Geometry check sheet. Reference: the model listing, model coordinates, mm. Face numbers are marked on the shaded views. A direction names the side the tool comes from. Coordinates: 2 decimals unless noted, no trailing zeros. Loops run counter-clockwise (first coordinate to the right, second up) from the corner with the lowest first, then second, coordinate; pieces in that order, holes last. Notation, with made-up numbers: M 1.25,39 L 20.25,39 A13 cw 20.25,60 Z; hole C 50,-27 d4. An arc over 180 degrees is marked long. One line per question, with ' | ' between items. Start each with the question number.
from build123d import *

# Parameters (mm, degrees)
F1_DEPTH = 18
F2_DEPTH = 16
F3_DEPTH = 14
F4_DEPTH = 12
F5_DEPTH = 10
F6_DEPTH = 8
F7_DEPTH = 6
F8_DEPTH = 4
F9_DEPTH = 2


with BuildPart() as f1:
    # F0 (on Top) → F1 (new body)
    with BuildSketch(Plane.XY):
        with BuildLine():
            Line((-5, 0), (-4.5, 0))
            ThreePointArc((-4.5, 0), (0, 4.5), (4.5, 0))
            Line((4.5, 0), (5, 0))
            ThreePointArc((5, 0), (0, 5), (-5, 0))
        make_face()
    extrude(amount=F1_DEPTH)

    # F0 (on Top) → F2 (join)
    with BuildSketch(Plane.XY):
        with BuildLine():
            Line((-4.5, 0), (-4, 0))
            ThreePointArc((-4, 0), (0, 4), (4, 0))
            Line((4, 0), (4.5, 0))
            ThreePointArc((4.5, 0), (0, 4.5), (-4.5, 0))
        make_face()
    extrude(amount=F2_DEPTH)

    # F0 (on Top) → F3 (join)
    with BuildSketch(Plane.XY):
        with BuildLine():
            Line((-4, 0), (-3.5, 0))
            ThreePointArc((-3.5, 0), (0, 3.5), (3.5, 0))
            Line((3.5, 0), (4, 0))
            ThreePointArc((4, 0), (0, 4), (-4, 0))
        make_face()
    extrude(amount=F3_DEPTH)

    # F0 (on Top) → F4 (join)
    with BuildSketch(Plane.XY):
        with BuildLine():
            Line((-3.5, 0), (-3, 0))
            ThreePointArc((-3, 0), (0, 3), (3, 0))
            Line((3, 0), (3.5, 0))
            ThreePointArc((3.5, 0), (0, 3.5), (-3.5, 0))
        make_face()
    extrude(amount=F4_DEPTH)

    # F0 (on Top) → F5 (join)
    with BuildSketch(Plane.XY):
        with BuildLine():
            Line((-3, 0), (-2.5, 0))
            ThreePointArc((-2.5, 0), (0, 2.5), (2.5, 0))
            Line((2.5, 0), (3, 0))
            ThreePointArc((3, 0), (0, 3), (-3, 0))
        make_face()
    extrude(amount=F5_DEPTH)

    # F0 (on Top) → F6 (join)
    with BuildSketch(Plane.XY):
        with BuildLine():
            Line((-2.5, 0), (-2, 0))
            ThreePointArc((-2, 0), (0, 2), (2, 0))
            Line((2, 0), (2.5, 0))
            ThreePointArc((2.5, 0), (0, 2.5), (-2.5, 0))
        make_face()
    extrude(amount=F6_DEPTH)

    # F0 (on Top) → F7 (join)
    with BuildSketch(Plane.XY):
        with BuildLine():
            Line((-2, 0), (-1.5, 0))
            ThreePointArc((-1.5, 0), (0, 1.5), (1.5, 0))
            Line((1.5, 0), (2, 0))
            ThreePointArc((2, 0), (0, 2), (-2, 0))
        make_face()
    extrude(amount=F7_DEPTH)

    # F0 (on Top) → F8 (join)
    with BuildSketch(Plane.XY):
        with BuildLine():
            Line((-1.5, 0), (-1, 0))
            ThreePointArc((-1, 0), (0, 1), (1, 0))
            Line((1, 0), (1.5, 0))
            ThreePointArc((1.5, 0), (0, 1.5), (-1.5, 0))
        make_face()
    extrude(amount=F8_DEPTH)

    # F0 (on Top) → F9 (join)
    with BuildSketch(Plane.XY):
        with BuildLine():
            Line((-1, 0), (-0.5, 0))
            ThreePointArc((-0.5, 0), (0, 0.5), (0.5, 0))
            Line((0.5, 0), (1, 0))
            ThreePointArc((1, 0), (0, 1), (-1, 0))
        make_face()
    extrude(amount=F9_DEPTH)

    # F10 (on Front) → F11 (revolve, cut)
    with BuildSketch(Plane.XZ):
        Polygon((5, 17.103553), (4.75, 17), (5, 16.896447), align=None)
        Polygon((4.75, 16), (5, 15.896447), (5, 16.103553), align=None)
        Polygon((4.75, 15), (5, 14.896447), (5, 15.103553), align=None)
        Polygon((4.75, 14), (5, 13.896447), (5, 14.103553), align=None)
        Polygon((4.75, 13), (5, 12.896447), (5, 13.103553), align=None)
        Polygon((4.75, 12), (5, 11.896447), (5, 12.103553), align=None)
        Polygon((4.75, 11), (5, 10.896447), (5, 11.103553), align=None)
        Polygon((4.75, 10), (5, 9.896447), (5, 10.103553), align=None)
        Polygon((4.75, 9), (5, 8.896447), (5, 9.103553), align=None)
        Polygon((4.75, 8), (5, 7.896447), (5, 8.103553), align=None)
        Polygon((4.75, 7), (5, 6.896447), (5, 7.103553), align=None)
        Polygon((4.75, 1), (5, 0.896447), (5, 1.103553), align=None)
        Polygon((4.75, 2), (5, 1.896447), (5, 2.103553), align=None)
        Polygon((4.75, 3), (5, 2.896447), (5, 3.103553), align=None)
        Polygon((4.75, 4), (5, 3.896447), (5, 4.103553), align=None)
        Polygon((4.75, 5), (5, 4.896447), (5, 5.103553), align=None)
        Polygon((4.75, 6), (5, 5.896447), (5, 6.103553), align=None)
    revolve(axis=Axis((5, 0, 9), (0, 0, 1)), mode=Mode.SUBTRACT)


solid = f1.part
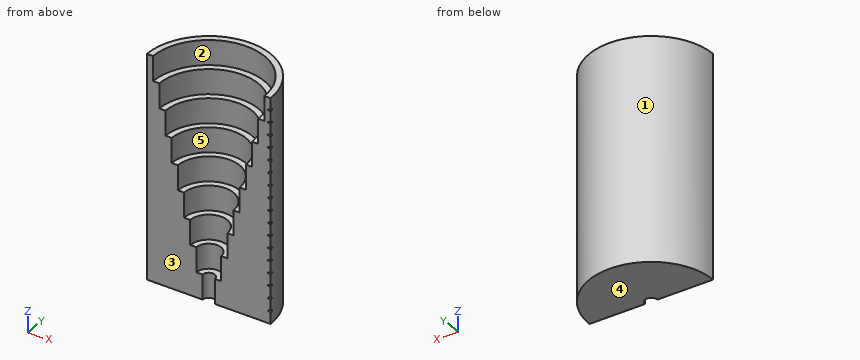
1. Sectioned sample at D-D (x = 3.25). Record the cut outline in (y, z).
2. Depth check by flat-ended pin: pin 1 Ø1.2 at (x, y) = (-0.5, 1) entering from +Z; pin 2 Ø4 at (x, z) = (0.5, 12) entering from +Y; pin 3 Ø1.5 at (y, z) = (4, 3) entering from -X; pin 4 Ø0.6 at (x, y) = (0.5, 1) entering from +Z. Enter the tip coordinate at first touch or a pass-through.
3. Thickness scan on line 1 (Z direction, x = -1.5, y = 1.9); line 2 (X direction, y = 1.9, z = 12.75); line 3 (Y direction, x = 4, z = 10). Record the ranges inside material, lowest first.
4. Draft check along X on the marked faces 1, 2 and 3. Enter one of: +X half, -X half, draft (parallel to the pull), parting line (faces both ways), or undercut.
5. Tool access check on the marked faces 4 and 5. Record the directions out of +Z, -Z, +X, -X, +Y, -Y that give a thin tool (end or side, any length) a straight path to the whole face; none if there is none.
6. Sectioned sample at C-C (z = 13.5). Record the cut outline in (x, y), and give its area (3 significant figures).
7. Sectioned sample at A-A (x = 0). Record the cut outline in (y, z).
Result:
1) outline: M 0,0 L 3.8,0 L 3.8,18 L 3.11,18 L 3.11,16 L 2.33,16 L 2.33,14 L 1.3,14 L 1.3,12 L 0,12 Z
2) pin 1: stops at z = 6 | pin 2: stops at y = 5 | pin 3: stops at x = -3.8 | pin 4: stops at z = 4
3) line 1: z = 0 to 8 | line 2: x = -4.62 to -2.94, 2.94 to 4.62 | line 3: y = 0 to 3
4) face 1: parting line | face 2: undercut | face 3: draft
5) face 4: -Z, +X, -X, +Y, -Y | face 5: +Z, -Y
6) outline: M -5,0 L -3.5,0 A3.5 cw 3.5,0 L 5,0 A5 ccw Z | area: 20.0 mm2
7) outline: M 0.5,0 L 5,0 L 5,18 L 4.5,18 L 4.5,16 L 4,16 L 4,14 L 3.5,14 L 3.5,12 L 3,12 L 3,10 L 2.5,10 L 2.5,8 L 2,8 L 2,6 L 1.5,6 L 1.5,4 L 1,4 L 1,2 L 0.5,2 Z
